Geometry check sheet. Reference: the model listing, model coordinates, mm. Round coordinates to 2 decimals unless told otherwise and drop trailing zeros. Order: outer loops, then holes, each group sorted by start corner. A loop starts at its lowest first (then second) coordinate and runs counter-clockwise, first axis right, second up. Notation, with made-up numbers: (47, -4.5) - (94, -4.5) arc R20 cw to (94, 19.5) - close; hole circle Ø7 at (89.25, -3). An arc over 180 degrees is marked (long way). Use a Markdown table: item, result. Add a question column.
(1) Thickness scan on line 1 along Y through (x, z) = (51, 0.35); line 2 along Y through (x, z) = (-37, 0.35); line 3 along X through (y, z) = (-97.5, 0.15). Record the ranges inside material, lowest first. Write a range as [from, to].
(2) Section check A-A on y = -126. Record the boundary of the cut face in (x, z).
(3) Mould release check, pull along Y, two halves, no side actions. Record for faces 1 (the face through (42, -111, 2)), 2 (the face through (39.638, -91.569, 0.986)): released by +Y, released by -Y, zero draft, split by the parting line, or undercut.
(4) Section check B-B on x = -5. Record the boundary of the cut face in (y, z), then the cut area to 3 significant figures.
(5) Section check C-C on y = -102.5. Record the boundary of the cut face in (x, z).
(6) Section check D-D on z = 1. Give the number of separate pieces and of enclosed holes in the cut face, then the cut area to 3 significant figures.
```python
from build123d import *

# Parameters (mm, degrees)
SKETCH_1_R          = 1.5
SKETCH_1_R_2        = 3.121318996
SKETCH_1_W          = 5.05
SKETCH_1_H          = 2.05
SKETCH_1_W_2        = 2.05
SKETCH_1_H_2        = 5.05
EXTRUDE_1_DEPTH     = 2
SKETCH_2_W          = 59.515578234
SKETCH_2_H          = 42.494416296
CUT_EXTRUDE_1_DEPTH = 10


with BuildPart() as part:
    # 草图1 → 凸台-拉伸1 (new body)
    with BuildSketch(Plane.XY):
        Polygon((-56.111334712, -13.372248853), (31.071025228, -13.372248853), (31.071025228, -137.372248853), (-56.111334712, -137.372248853), (-56.111334712, -152.372248853), (-56.111334712, -227.397248853), (62.919821756, -227.397248853), (62.919821756, -152.372248853), (62.919821756, 1.627751147), (-56.111334712, 1.627751147), align=None)
        with Locations((-19.586334712, -1.372248853)):
            Circle(SKETCH_1_R, mode=Mode.SUBTRACT)
        with Locations((20.413665288, -1.372248853)):
            Circle(SKETCH_1_R, mode=Mode.SUBTRACT)
        with Locations((-19.586334712, -149.372248853)):
            Circle(SKETCH_1_R, mode=Mode.SUBTRACT)
        with Locations((20.413665288, -149.372248853)):
            Circle(SKETCH_1_R, mode=Mode.SUBTRACT)
        with Locations((59.919821756, -97.372248853)):
            Circle(SKETCH_1_R, mode=Mode.SUBTRACT)
        with Locations((59.919821756, -57.372248853)):
            Circle(SKETCH_1_R, mode=Mode.SUBTRACT)
        with Locations((41.938665288, -93.678088908)):
            Circle(SKETCH_1_R_2, mode=Mode.SUBTRACT)
        with Locations((-19.586334712, -224.372248853)):
            Circle(SKETCH_1_R, mode=Mode.SUBTRACT)
        with Locations((20.413665288, -224.372248853)):
            Circle(SKETCH_1_R, mode=Mode.SUBTRACT)
        with Locations((39.413665288, -1.372248853)):
            Rectangle(SKETCH_1_W, SKETCH_1_H, mode=Mode.SUBTRACT)
        with Locations((49.413665288, -1.372248853)):
            Rectangle(SKETCH_1_W, SKETCH_1_H, mode=Mode.SUBTRACT)
        with Locations((-48.586334712, -1.372248853)):
            Rectangle(SKETCH_1_W, SKETCH_1_H, mode=Mode.SUBTRACT)
        with Locations((-38.586334712, -1.372248853)):
            Rectangle(SKETCH_1_W, SKETCH_1_H, mode=Mode.SUBTRACT)
        with Locations((39.413665288, -149.372248853)):
            Rectangle(SKETCH_1_W, SKETCH_1_H, mode=Mode.SUBTRACT)
        with Locations((49.413665288, -149.372248853)):
            Rectangle(SKETCH_1_W, SKETCH_1_H, mode=Mode.SUBTRACT)
        with Locations((-48.586334712, -149.372248853)):
            Rectangle(SKETCH_1_W, SKETCH_1_H, mode=Mode.SUBTRACT)
        with Locations((-38.586334712, -149.372248853)):
            Rectangle(SKETCH_1_W, SKETCH_1_H, mode=Mode.SUBTRACT)
        with Locations((59.919821756, -38.372248853)):
            Rectangle(SKETCH_1_W_2, SKETCH_1_H_2, mode=Mode.SUBTRACT)
        with Locations((59.919821756, -28.372248853)):
            Rectangle(SKETCH_1_W_2, SKETCH_1_H_2, mode=Mode.SUBTRACT)
        with Locations((59.919821756, -126.372248853)):
            Rectangle(SKETCH_1_W_2, SKETCH_1_H_2, mode=Mode.SUBTRACT)
        with Locations((59.919821756, -116.372248853)):
            Rectangle(SKETCH_1_W_2, SKETCH_1_H_2, mode=Mode.SUBTRACT)
        with Locations((39.413665288, -224.372248853)):
            Rectangle(SKETCH_1_W, SKETCH_1_H, mode=Mode.SUBTRACT)
        with Locations((49.413665288, -224.372248853)):
            Rectangle(SKETCH_1_W, SKETCH_1_H, mode=Mode.SUBTRACT)
        with Locations((-48.586334712, -224.372248853)):
            Rectangle(SKETCH_1_W, SKETCH_1_H, mode=Mode.SUBTRACT)
        with Locations((-38.586334712, -224.372248853)):
            Rectangle(SKETCH_1_W, SKETCH_1_H, mode=Mode.SUBTRACT)
    extrude(amount=EXTRUDE_1_DEPTH)

    # 草图2 → 切除-拉伸1 (cut)
    with BuildSketch(Plane.XY.offset(2)):
        with Locations((-26.353545595, -206.150040705)):
            Rectangle(SKETCH_2_W, SKETCH_2_H)
    extrude(amount=-CUT_EXTRUDE_1_DEPTH, mode=Mode.SUBTRACT)


solid = part.part
```
Check sheet entries:
| question | item | result |
|---|---|---|
| 1 | line 1 | y = [-227.4, -225.4], [-223.35, -150.4], [-148.35, -2.4], [-0.35, 1.63] |
| 1 | line 2 | y = [-184.9, -150.4], [-148.35, -137.37], [-13.37, -2.4], [-0.35, 1.63] |
| 1 | line 3 | x = [31.07, 58.43], [61.41, 62.92] |
| 2 | outline | (31.07, 0) - (58.89, 0) - (58.89, 2) - (31.07, 2) - close; (60.94, 0) - (62.92, 0) - (62.92, 2) - (60.94, 2) - close |
| 3 | face 1 | zero draft |
| 3 | face 2 | undercut |
| 4 | outline | (-184.9, 0) - (-137.37, 0) - (-137.37, 2) - (-184.9, 2) - close; (-13.37, 0) - (1.63, 0) - (1.63, 2) - (-13.37, 2) - close |
| 4 | area | 125 mm2 |
| 5 | outline | (31.07, 0) - (62.92, 0) - (62.92, 2) - (31.07, 2) - close |
| 6 | separate pieces | 1 |
| 6 | enclosed holes | 22 |
| 6 | area | 13,700 mm2 |
